from build123d import *

# Parameters (mm, degrees)
F0_R     = 15.920661
F1_DEPTH = 25.4
F2_DEPTH = 6.35
F4_DEPTH = 19.05
F6_DEPTH = 1752.6


with BuildPart() as f1:
    # F0 (on Top) → F1 (new body)
    with BuildSketch(Plane.XY):
        with BuildLine():
            ThreePointArc((-31.421627, 24.693735), (-38.573704, 27.846859), (-46.308367, 28.973528))
            ThreePointArc((-46.308367, 28.973528), (-75.554202, 0), (-46.308367, -28.973528))
            ThreePointArc((-46.308367, -28.973528), (-37.375926, -27.474257), (-29.342811, -23.290312))
            ThreePointArc((-29.342811, -23.290312), (-17.631762, 1.2541), (-31.421627, 24.693735))
        make_face()
        with Locations((-46.579406, 0)):
            Circle(F0_R, mode=Mode.SUBTRACT)
    extrude(amount=F1_DEPTH)

    # F0 (on Top) → F2 (join)
    with BuildSketch(Plane.XY):
        with BuildLine():
            Line((30.658745, 24.693735), (-31.421627, 24.693735))
            ThreePointArc((-31.421627, 24.693735), (-17.631762, 1.2541), (-29.342811, -23.290312))
            Line((-29.342811, -23.290312), (30.658745, -23.290312))
            Line((30.658745, -23.290312), (30.658745, 0))
            Line((30.658745, 0), (30.658745, 24.693735))
        make_face()
    extrude(amount=F2_DEPTH)

    # F3 (on face) → F4 (join)
    with BuildSketch(Plane.XY.offset(6.35)):
        with BuildLine():
            Line((16.550291, 4.09937), (-17.896066, 4.09937))
            ThreePointArc((-17.896066, 4.09937), (-17.604695, 0.070426), (-17.876477, -3.959886))
            Line((-17.876477, -3.959886), (16.550291, -3.959886))
            Line((16.550291, -3.959886), (16.550291, 4.09937))
        make_face()
    extrude(amount=F4_DEPTH)

    # F5 (on face) → F6 (cut)
    with BuildSketch(Plane.XZ.offset(3.959886)):
        Polygon((16.550291, 25.4), (-17.876477, 25.4), (16.550291, 6.35), align=None)
    extrude(amount=-F6_DEPTH, mode=Mode.SUBTRACT)


solid = f1.part
Design review of the part built by this model. Coordinates are the model's own, in mm. A direction names the side the tool comes from. Round coordinates to 2 decimals unless told otherwise and drop trailing zeros. Write each loop counter-clockwise with the first axis right and the second up, starting at its lowest first coordinate (ties: lowest second). Pieces come first, ordered by that corner, then holes. Notation, with made-up numbers: (18.5, 67.25) - (40.5, 67.25) arc R11 ccw to (40.5, 74.25) - close; hole circle Ø6 at (86.25, 51.25). An arc over 180 degrees is marked (long way). Return JSON: item names as keys, results as strings. Group by question number.
Item 1: Machinability: for faces 4 (the face through (-4, 4.099, 14)), 5 (the face through (-5, -3.96, 14)), 6 (the face through (0, -23.29, 3)), which of the approach directions +Z, -Z, +X, -X, +Y, -Y give a long, thin tool a straight path to every point of the face, cutting with its end or side? Answer none if there is none.
Item 2: We need section D-D on x = -37. Write out the cut boundary in (y, z).
Item 3: The part is to be moulded in two halves that separate along X. For faces 1 (the face through (-59.21, -9.69, 12.52)), 2 (the face through (-0.904, 0.013, 16.008)), 3 (the face through (6, 6, 6.35)), say which applies: pulls with the +X half, pulls with the -X half, needs draft (parallel to the pull), parting line crosses it, or undercut.
Item 4: We need section A-A on y = 0. Write out the cut boundary in (x, z).
Item 5: We need section B-B on x = -50.5. Write out the cut boundary in (y, z), and give its area (3 significant figures).
Item 6: For probe 1 along Z at (x, y) = (13, 19); probe 2 along Y at (x, z) = (-3.5, 9.75); probe 3 along Y at (x, z) = (-61, 10), list the stretches that pass through material, from the lowest coordinate up. Write a range as [from, to].
Item 7: Insertion check: P1, Ø6, axis at y = -20.5, z = 10.5, coming from the -X side; P2, Ø9.5, axis at x = 4.5, z = 11, coming from the +Y side; P3, Ø3, axis at y = 4.5, z = 21.5, coming from the +X side. Each pin has a flat end and moves straight along its axis. Give the tip position at first contact, or say it passes through.
Model answer:
{
 "1": {"face 4": "+Z, +X, +Y", "face 5": "+Z, +X, -Y", "face 6": "+Z, -Z, +X, -Y"},
 "2": {"outline": "(-27.35, 0) - (-12.72, 0) - (-12.72, 25.4) - (-27.35, 25.4) - close; (12.72, 0) - (27.35, 0) - (27.35, 25.4) - (12.72, 25.4) - close"},
 "3": {"face 1": "undercut", "face 2": "pulls with the +X half", "face 3": "needs draft"},
 "4": {"outline": "(-75.55, 0) - (-62.5, 0) - (-62.5, 25.4) - (-75.55, 25.4) - close; (-30.66, 0) - (30.66, 0) - (30.66, 6.35) - (16.55, 6.35) - (-17.88, 25.4) - (-30.66, 25.4) - close"},
 "5": {"outline": "(-28.71, 0) - (-15.43, 0) - (-15.43, 25.4) - (-28.71, 25.4) - close; (15.43, 0) - (28.71, 0) - (28.71, 25.4) - (15.43, 25.4) - close", "area": "675 mm²"},
 "6": {"probe 1": "z = [0, 6.35]", "probe 2": "y = [-3.96, 4.1]", "probe 3": "y = [-25.13, -6.75], [6.75, 25.13]"},
 "7": {"P1": "stops at x = -69.67", "P2": "stops at y = 24.69", "P3": "stops at x = -8.22"}
}
